from build123d import *

# Parameters (mm, degrees)
SKETCH1_R           = 9
EXTRUDE1_DEPTH      = 212.5
CHAMFER1_SIZE       = 1.35
SKETCH3_W           = 6
SKETCH3_H           = 3.5
EXTRUDE2_DEPTH      = 213.5
EXTRUDE2_DEPTH_BACK = 213.5


with BuildPart() as part:
    # Sketch1 → Extrude1 (new body, symmetric)
    with BuildSketch(Plane.XY):
        Circle(SKETCH1_R)
    extrude(amount=EXTRUDE1_DEPTH, both=True)

    # Chamfer1
    chamfer1_edges = [part.edges().sort_by_distance(p)[0] for p in [
        (-9, 0, -212.5),
        (-9, 0, 212.5),
    ]]
    chamfer(chamfer1_edges, length=CHAMFER1_SIZE)

    # Sketch3 → Extrude2 (cut, two sides)
    with BuildSketch(Plane.XY) as extrude2_sk:
        with Locations((0, 7.25)):
            Rectangle(SKETCH3_W, SKETCH3_H)
    extrude(amount=EXTRUDE2_DEPTH, mode=Mode.SUBTRACT)
    extrude(extrude2_sk.sketch, amount=-EXTRUDE2_DEPTH_BACK, mode=Mode.SUBTRACT)


solid = part.part
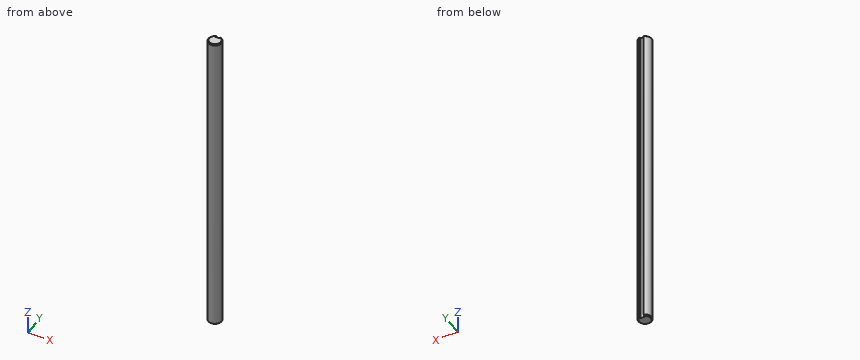
Design review of the part built by this model. Coordinates are the model's own, in mm. Coordinates: 2 decimals unless noted, no trailing zeros. Order: outer loops, then holes, each group sorted by start corner. A loop starts at its lowest first (then second) coordinate and runs counter-clockwise, first axis right, second up. Notation, with made-up numbers: (40.5, 59.5) -> (87.5, 59.5) arc R18 cw to (87.5, 67.5) -> close; hole circle Ø1 at (65.25, 70). An arc over 180 degrees is marked (long way). Use one line per item in the form item = value. Start each with the question number.
(1) Add section A-A on x = 0. State the section outline as (y, z) points.
(2) Insertion check: pin 1 (3 mm diameter, centred on x = -2.5, z = -104.5, fed in from -Y); pin 2 (3.5 mm diameter, centred on y = 6.5, z = -94.5, fed in from -X); pin 3 (4 mm diameter, centred on y = -6.5, z = 167.5, fed in from +X). Each pin has a flat end and moves straight along its axis. Give the tip position at first contact, or say it passes through.
(3) For probe 1 along X at (y, z) = (-1, -180.5); probe 2 along Y at (x, z) = (1, -102); probe 3 along Y at (x, z) = (0.75, 128), list the stretches that pass through material, from the lowest coordinate up.
(4) Add section B-B on z = 145. State the section outline as (x, y) points.
Answer block:
q1.outline = (-9, -211.15) -> (-7.65, -212.5) -> (5.5, -212.5) -> (5.5, 212.5) -> (-7.65, 212.5) -> (-9, 211.15) -> close
q2.pin_1 = -8.94
q2.pin_2 = -7.64
q2.pin_3 = 7.79
q3.probe_1 = -8.94 to 8.94
q3.probe_2 = -8.94 to 5.5
q3.probe_3 = -8.97 to 5.5
q4.outline = (-3, 5.5) -> (-3, 8.49) arc R9 ccw (long way) to (3, 8.49) -> (3, 5.5) -> close
